from build123d import *

# Parameters (mm, degrees)
F0_W      = 18
F0_H      = 18
F1_DEPTH  = 18
F2_W      = 12.4
F2_H      = 12.4
F3_DEPTH  = 4
F4_DEPTH  = 4
F5_W      = 6.2
F5_H      = 12.4
F6_DEPTH  = 4
F7_W      = 6.2
F7_H      = 12.4
F8_DEPTH  = 4
F9_W      = 6.2
F9_H      = 12.4
F10_DEPTH = 4
F11_W     = 6.2
F11_H     = 12.4
F12_DEPTH = 4


with BuildPart() as f1:
    # F0 (on Top) → F1 (new body)
    with BuildSketch(Plane.XY):
        Rectangle(F0_W, F0_H)
    extrude(amount=F1_DEPTH)

    # F2 (on face) → F3 (join)
    with BuildSketch(Plane.XY.offset(18)):
        Rectangle(F2_W, F2_H)
    extrude(amount=F3_DEPTH)

    # F2 (on face) → F4 (join)
    with BuildSketch(Plane.XY.offset(18)):
        Rectangle(F2_W, F2_H)
    extrude(amount=-F4_DEPTH)

    # F5 (on face) → F6 (join)
    with BuildSketch(Plane(origin=(0, 9, 0), x_dir=(-1, 0, 0), z_dir=(0, 1, 0))):
        with Locations((3.1, 9)):
            Rectangle(F5_W, F5_H)
        with Locations((-3.1, 9)):
            Rectangle(F5_W, F5_H)
    extrude(amount=F6_DEPTH)

    # F7 (on face) → F8 (join)
    with BuildSketch(Plane(origin=(-9, 0, 0), x_dir=(0, -1, 0), z_dir=(-1, 0, 0))):
        with Locations((3.1, 9)):
            Rectangle(F7_W, F7_H)
        with Locations((-3.1, 9)):
            Rectangle(F7_W, F7_H)
    extrude(amount=F8_DEPTH)

    # F9 (on face) → F10 (join)
    with BuildSketch(Plane.YZ.offset(9)):
        with Locations((3.1, 9)):
            Rectangle(F9_W, F9_H)
        with Locations((-3.1, 9)):
            Rectangle(F9_W, F9_H)
    extrude(amount=F10_DEPTH)

    # F11 (on face) → F12 (join)
    with BuildSketch(Plane.XZ.offset(9)):
        with Locations((3.1, 9)):
            Rectangle(F11_W, F11_H)
        with Locations((-3.1, 9)):
            Rectangle(F11_W, F11_H)
    extrude(amount=F12_DEPTH)


solid = f1.part
Model file for the job. Use its own axes, mm. A direction names the side the tool comes from. Give positions to 0.01 mm unless a question says otherwise; leave off trailing zeros. Write each loop counter-clockwise with the first axis right and the second up, starting at its lowest first coordinate (ties: lowest second). Pieces come first, ordered by that corner, then holes. Notation, with made-up numbers: M -15.75,6.25 L 12.25,6.25 A21 cw 12.25,29.25 Z; hole C 38,68.25 d7. An arc over 180 degrees is marked long. One line per item, written item: value. Start each with the question number.
Q1. Probe probe 1 along Z at (x, y) = (-4.5, -7.5); probe 2 along X at (y, z) = (-7, 12.25); probe 3 along Y at (x, z) = (-5.75, 20.75). List the from-to ranges inside material, lowest first. Write a range as [from, to].
Q2. 3-axis set-ups, long thin cutter, end or side, ignore diameter. For faces 1 (the flat face through (11, 0, 2.8)), 2 (the flat face through (-11, 0, 15.2)), 3 (the flat face through (-11, 0, 2.8)), 4 (the flat face through (6.2, 0, 20)), 5 (the flat face through (6.2, 11, 9)): which of +Z, -Z, +X, -X, +Y, -Y reach the whole face in a straight line?
Q3. Saw through at B-B, the plane x = -3. Write the cut outline in (y, z), plus the area to 3 significant figures.
Q4. Saw through at D-D, the plane z = 20.75. Write the cut outline in (x, y).
Q5. Drop flat-ended pins along their axis: pin 1 Ø3 at (x, y) = (-0.5, -11) entering from +Z; pin 2 Ø3 at (y, z) = (-11, 8) entering from +X; pin 3 Ø3 at (x, z) = (-10, 7.5) entering from +Y; pin 4 Ø3 at (x, y) = (-3, 7) entering from +Z. Give the stop position or say it passes through.
Q6. Saw through at A-A, the plane z = 10.5. Write the cut outline in (x, y).
Output values:
1. probe 1: z = [0, 18]
1. probe 2: x = [-9, 9]
1. probe 3: y = [-6.2, 6.2]
2. face 1: -Z, +X, +Y, -Y
2. face 2: +Z, -X, +Y, -Y
2. face 3: -Z, -X, +Y, -Y
2. face 4: +Z, +X, +Y, -Y
2. face 5: +Z, -Z, +X, +Y
3. outline: M -13,2.8 L -9,2.8 L -9,0 L 9,0 L 9,2.8 L 13,2.8 L 13,15.2 L 9,15.2 L 9,18 L 6.2,18 L 6.2,22 L -6.2,22 L -6.2,18 L -9,18 L -9,15.2 L -13,15.2 Z
3. area: 473 mm²
4. outline: M -6.2,-6.2 L 6.2,-6.2 L 6.2,6.2 L -6.2,6.2 Z
5. pin 1: stops at z = 15.2
5. pin 2: stops at x = 6.2
5. pin 3: stops at y = 9
5. pin 4: stops at z = 22
6. outline: M -13,-6.2 L -9,-6.2 L -9,-9 L -6.2,-9 L -6.2,-13 L 6.2,-13 L 6.2,-9 L 9,-9 L 9,-6.2 L 13,-6.2 L 13,6.2 L 9,6.2 L 9,9 L 6.2,9 L 6.2,13 L -6.2,13 L -6.2,9 L -9,9 L -9,6.2 L -13,6.2 Z
